```python
from build123d import *

# Parameters (mm, degrees)
BOSS_EXTRUDE1_DEPTH = 30
SKETCH2_W           = 10
SKETCH2_H           = 26
CUT_EXTRUDE1_DEPTH  = 5
SKETCH3_R           = 5
BOSS_EXTRUDE2_DEPTH = 1
SKETCH4_R           = 7.5
BOSS_EXTRUDE3_DEPTH = 1
SKETCH5_R           = 5
BOSS_EXTRUDE4_DEPTH = 1


with BuildPart() as part:
    # Sketch1 → Boss-Extrude1 (new body)
    with BuildSketch(Plane.XY):
        Polygon((-10.17985471, 6.184971098), (-10.17985471, -8.815028902), (-5.17985471, -8.815028902), (-5.17985471, -4.815028902), (14.82014529, -4.815028902), (14.82014529, 0.184971098), (-5.17985471, 0.184971098), (-5.17985471, 6.184971098), align=None)
    extrude(amount=BOSS_EXTRUDE1_DEPTH)

    # Sketch2 → Cut-Extrude1 (cut)
    with BuildSketch(Plane(origin=(0, 0.184971098, 0), x_dir=(1, 0, 0), z_dir=(0, 1, 0))):
        with Locations((2.82014529, -15)):
            Rectangle(SKETCH2_W, SKETCH2_H)
    extrude(amount=-CUT_EXTRUDE1_DEPTH, mode=Mode.SUBTRACT)

    # Sketch3 → Boss-Extrude2 (add)
    with BuildSketch(Plane.ZY.offset(10.17985471)):
        with Locations((15, -1.315028902)):
            Circle(SKETCH3_R)
    extrude(amount=BOSS_EXTRUDE2_DEPTH)

    # Sketch4 → Boss-Extrude3 (add)
    with BuildSketch(Plane.ZY.offset(11.17985471)):
        with Locations((15, -1.315028902)):
            Circle(SKETCH4_R)
    extrude(amount=BOSS_EXTRUDE3_DEPTH)

    # Sketch5 → Boss-Extrude4 (add)
    with BuildSketch(Plane.ZY.offset(12.17985471)):
        with Locations((15, -1.315028902)):
            Circle(SKETCH5_R)
    extrude(amount=BOSS_EXTRUDE4_DEPTH)


solid = part.part
```
Model file for the job. Use its own axes, mm. A direction names the side the tool comes from. Round coordinates to 2 decimals unless told otherwise and drop trailing zeros. Write each loop counter-clockwise with the first axis right and the second up, starting at its lowest first coordinate (ties: lowest second). Pieces come first, ordered by that corner, then holes. Notation, with made-up numbers: M 54,9 L 84,9 A10 ccw 84,13 Z; hole C -3.5,-23 d11. An arc over 180 degrees is marked long. Put each result on its own line as item: value.
Item 1: Cut at B-B (y = 4.25). List the corners of the cut face in (x, z).
Responses:
outline: M -12.18,9.97 L -11.18,9.97 L -11.18,20.03 L -12.18,20.03 Z; M -10.18,0 L -5.18,0 L -5.18,30 L -10.18,30 Z
Item 2: Cut at A-A (z = 15). List the corners of the cut face in (x, y), and give its area (3 significant figures).
Responses:
outline: M -13.18,-6.32 L -12.18,-6.32 L -12.18,-8.82 L -11.18,-8.82 L -11.18,-6.32 L -10.18,-6.32 L -10.18,-8.82 L -5.18,-8.82 L -5.18,-4.82 L -2.18,-4.82 L -2.18,0.18 L -5.18,0.18 L -5.18,6.18 L -10.18,6.18 L -10.18,3.68 L -11.18,3.68 L -11.18,6.18 L -12.18,6.18 L -12.18,3.68 L -13.18,3.68 Z; M 7.82,-4.82 L 14.82,-4.82 L 14.82,0.18 L 7.82,0.18 Z
area: 160 mm²
Item 3: Tool access for faces 1 (the flat face through (7.82, -2, 15)), 2 (the flat face through (-5.18, 3, 15)), 3 (the cylindrical face through (-10.67, 0.19, 19.77)): list every direction of +Z, -Z, +X, -X, +Y, -Y with a clear straight run to the whole face (end or side of a thin tool).
Responses:
face 1: +Y, -Y
face 2: +Z, -Z, +X, +Y
face 3: none
Item 4: Cut at C-C (z = 9). List the corners of the cut face in (x, y).
Responses:
outline: M -12.18,-5.82 L -11.18,-5.82 L -11.18,3.18 L -12.18,3.18 Z; M -10.18,-8.82 L -5.18,-8.82 L -5.18,-4.82 L -2.18,-4.82 L -2.18,0.18 L -5.18,0.18 L -5.18,6.18 L -10.18,6.18 Z; M 7.82,-4.82 L 14.82,-4.82 L 14.82,0.18 L 7.82,0.18 Z
Item 5: Mould opens along Z. For faces 4 (the flat face through (3, -2, 2)), 5 (the flat face through (-5.18, -7, 15)), 6 (the flat face through (-1, -3, 0)), 7 (the flat face through (-1, -3, 30)) say: +Z half, -Z half, draft (parallel to the pull), parting line (faces both ways), or undercut.
Responses:
face 4: undercut
face 5: draft
face 6: -Z half
face 7: +Z half
Item 6: Cut at D-D (y = -3). List the corners of the cut face in (x, z).
Responses:
outline: M -13.18,10.29 L -12.18,10.29 L -12.18,7.69 L -11.18,7.69 L -11.18,10.29 L -10.18,10.29 L -10.18,0 L 14.82,0 L 14.82,30 L -10.18,30 L -10.18,19.71 L -11.18,19.71 L -11.18,22.31 L -12.18,22.31 L -12.18,19.71 L -13.18,19.71 Z; hole M -2.18,2 L 7.82,2 L 7.82,28 L -2.18,28 Z
Item 7: Probe L1, parallel to X at y = -5.5, z = 10.5; L2, parallel to Z at x = -0.5, y = -2; L3, parallel to X at y = -0.5, z = 24.5. List the from-to ranges inside material, lowest first. Write a range as from..to.
Responses:
L1: -12.18..-11.18, -10.18..-5.18
L2: 0..2, 28..30
L3: -10.18..-2.18, 7.82..14.82
Item 8: Flat gauge pins, fed straight in: P1, Ø6, axis at x = 6.5, z = 15.5, coming from the -Y side (3 decimals); P2, Ø10, axis at x = 0.5, z = 7, coming from the +Y side (3 decimals); P3, Ø3, axis at y = 3.5, z = 15.5, coming from the +X side. Where does each tip first touch, or does it go through?
Responses:
P1: y = -4.815
P2: y = 0.185
P3: x = -5.18
